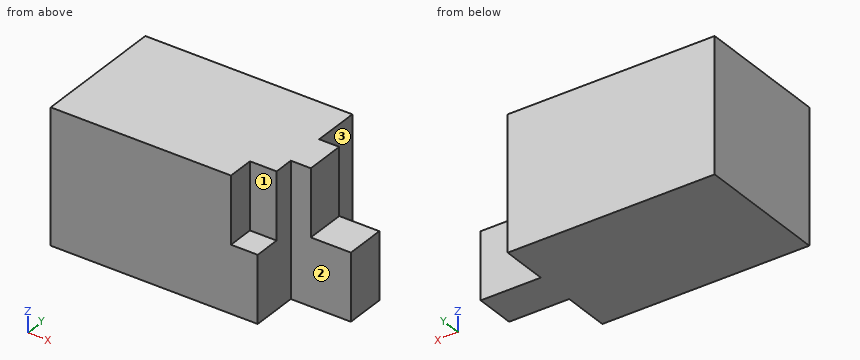
from build123d import *

# Parameters (mm, degrees)
F1_DEPTH = 25
F2_W     = 22.5
F2_H     = 17.5
F3_DEPTH = 50
F4_W     = 10
F4_H     = 10
F5_DEPTH = 25


with BuildPart() as f1:
    # F0 (on Front) → F1 (new body, symmetric)
    with BuildSketch(Plane.XZ):
        Polygon((35, 50), (-50, 50), (-50, 0), (50, 0), (50, 25), (35, 25), align=None)
    extrude(amount=F1_DEPTH, both=True)

    # F2 (on face) → F3 (cut, through all)
    with BuildSketch(Plane.XY.offset(50)):
        with Locations((38.75, 16.25)):
            Rectangle(F2_W, F2_H)
        with Locations((38.75, -16.25)):
            Rectangle(F2_W, F2_H)
    extrude(amount=-F3_DEPTH, mode=Mode.SUBTRACT)

    # F4 (on face) → F5 (cut)
    with BuildSketch(Plane.XY.offset(50)):
        with Locations((22.5, -20)):
            Rectangle(F4_W, F4_H)
    extrude(amount=-F5_DEPTH, mode=Mode.SUBTRACT)


solid = f1.part
Model file for the job. Use its own axes, mm. Face numbers are marked on the shaded views. A direction names the side the tool comes from. Round coordinates to 2 decimals unless told otherwise and drop trailing zeros. Order: outer loops, then holes, each group sorted by start corner. A loop starts at its lowest first (then second) coordinate and runs counter-clockwise, first axis right, second up.
(1) Band-saw the part on D-D (z = 19). List the corners of the cut face in (x, y).
(2) Band-saw the part on B-B (y = 0). List the corners of the cut face in (x, z).
(3) Band-saw the part on C-C (x = 30.5). List the corners of the cut face in (y, z), then the cut area to 3 significant figures.
(4) Band-saw the part on A-A (z = 33.5). List the corners of the cut face in (x, y).
(5) 3-axis set-ups, long thin cutter, end or side, ignore diameter. For the marked faces 1, 2 and 3: which of +Z, -Z, +X, -X, +Y, -Y reach the whole face in a straight line?
(6) Pin check, flat tips, straight feed: pin 1 (11 mm diameter, centred on x = 40, z = 16, fed in from +Y); pin 2 (7 mm diameter, centred on x = 40.5, z = 24, fed in from -Y); pin 3 (3 mm diameter, centred on y = -6, z = 31, fed in from +X); pin 4 (3 mm diameter, centred on x = 29.5, y = 15.5, fed in from +Z). Stop position of each tip, or through.
(7) Drill centre lines: line 1 (X direction, y = -9, z = 18.5); line 2 (X direction, y = 6.5, z = 33.5); line 3 (Z direction, x = 41, y = -6.5). Where is each one in solid material? Low to high.
Verdict:
1. outline: (-50, -25) - (27.5, -25) - (27.5, -7.5) - (50, -7.5) - (50, 7.5) - (27.5, 7.5) - (27.5, 25) - (-50, 25) - close
2. outline: (-50, 0) - (50, 0) - (50, 25) - (35, 25) - (35, 50) - (-50, 50) - close
3. outline: (-7.5, 0) - (7.5, 0) - (7.5, 50) - (-7.5, 50) - close
3. area: 750 mm2
4. outline: (-50, -25) - (17.5, -25) - (17.5, -15) - (27.5, -15) - (27.5, -7.5) - (35, -7.5) - (35, 7.5) - (27.5, 7.5) - (27.5, 25) - (-50, 25) - close
5. face 1: +Z, +X, -Y
5. face 2: +Z, -Z, +X, -Y
5. face 3: +Z, -Z, +X, +Y
6. pin 1: stops at y = 7.5
6. pin 2: stops at y = -7.5
6. pin 3: stops at x = 35
6. pin 4: passes through
7. line 1: x = -50 to 27.5
7. line 2: x = -50 to 35
7. line 3: z = 0 to 25
